Autodesk Inventor part; units mm, degrees
ref_plane "to_a_XY" through (0, 9.6037, 0) normal (0, 1, 0) x (1, 0, 0)
ref_plane "to_a_YZ" through (0, 9.6037, 0) normal (1, 0, 0) x (0, 0, -1)
ref_plane "to_a_ZX" through (0, 9.6037, 0) normal (0, 0, -1) x (0, 1, 0)
sketch "Sketch_1" plane through (0, 0, 0) normal (0, 0, 1) x (1, 0, 0)
  line L0 (0, 0) -> (0, 20.574)
  line L1 (0, 20.574) -> (2.6561, 20.574)
  arc A0 (5.5506, 18.0111) -> (2.6561, 20.574) centre (0.9891, 15.7753) ccw
  line L2 (5.5506, 18.0111) -> (5.5506, 17.2237)
  line L3 (5.5506, 17.2237) -> (2.3752, 17.2237)
  line L4 (2.3752, 17.2237) -> (2.3752, 10.414)
  line L5 (2.3752, 10.414) -> (3.175, 10.414)
  line L6 (3.175, 10.414) -> (3.175, 0.7557)
  line L7 (3.175, 0.7557) -> (2.4194, 0)
  line L8 (2.4194, 0) -> (0, 0)
  line L9 (0, 0) -> (0, 20.574)
revolve "Revolution1" add sketch "Sketch_1" angle 360 about axis through (0, 0, 0) along (0, -1, 0)
thread "Thread1"
sketch "Sketch_2" plane through (0, 20.574, 0) normal (0, 1, 0) x (1, 0, 0)
  line L0 (-7.62, 7.62) -> (-7.62, -7.62)
  line L1 (-7.62, -7.62) -> (7.62, -7.62)
  line L2 (7.62, -7.62) -> (7.62, 7.62)
  line L3 (7.62, 7.62) -> (-7.62, 7.62)
  line L4 (-2.3752, 6.35) -> (-2.3752, -6.35)
  line L5 (-2.3752, -6.35) -> (2.3752, -6.35)
  line L6 (2.3752, -6.35) -> (2.3752, 6.35)
  line L7 (2.3752, 6.35) -> (-2.3752, 6.35)
extrude "Extrusion1" cut sketch "Sketch_2" along normal mid plane 10.16
sketch "Sketch_3" plane through (0, 20.574, 0) normal (0, 1, 0) x (1, 0, 0)
  line L0 (-1.9814, -1.144) -> (0, -2.288)
  line L1 (0, -2.288) -> (1.9814, -1.144)
  line L2 (1.9814, -1.144) -> (1.9814, 1.144)
  line L3 (1.9814, 1.144) -> (0, 2.288)
  line L4 (0, 2.288) -> (-1.9814, 1.144)
  line L5 (-1.9814, 1.144) -> (-1.9814, -1.144)
extrude "Extrusion2" cut sketch "Sketch_3" against normal blind 2.2098
ref_plane "to_a_XY" through (0, 9.6037, 0) normal (0, 1, 0) x (1, 0, 0)
ref_plane "to_a_YZ" through (0, 9.6037, 0) normal (1, 0, 0) x (0, 0, -1)
ref_plane "to_a_ZX" through (0, 9.6037, 0) normal (0, 0, -1) x (0, 1, 0)
properties part number "2059_screw"
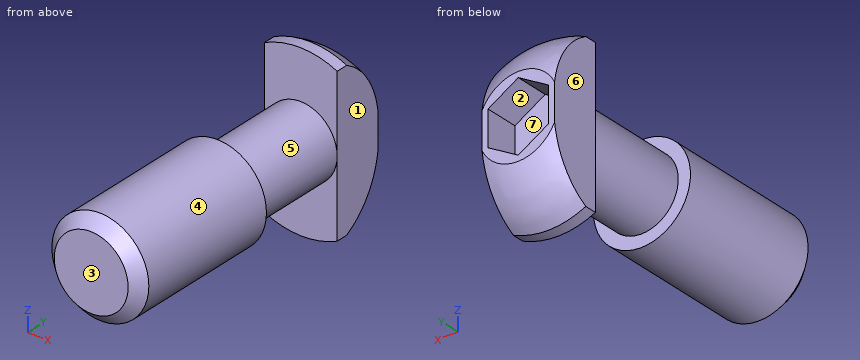
The listing builds one solid part. Answer for the finished solid, in the listing's coordinates (mm). Face numbers are marked on the shaded views. A direction names the side the tool comes from. Give positions to 0.01 mm unless a question says otherwise; leave off trailing zeros. Order: outer loops, then holes, each group sorted by start corner. A loop starts at its lowest first (then second) coordinate and runs counter-clockwise, first axis right, second up. Notation, with made-up numbers: (73.5, 74.5) - (88.5, 74.5) arc R19 cw to (88.5, 82.5) - close; hole circle Ø4 at (84.5, -9.75). An arc over 180 degrees is marked (long way). One line per item, written item: value. Start each with the question number.
1) A tool of negligible diameter and unlimited length cuts with its end or side. For the marked faces 1, 2, 3 and 4, from which of +Z, -Z, +X, -X, +Y, -Y can it reach the whole face along a straight path? Write none if from no direction.
2) Find the intervals of material crossed by L1, parallel to Y at x = 1.25, z = -1; L2, parallel to X at y = 17.5, z = -3.25; L3, parallel to Z at x = -1.5, y = 9.5, in increasing order.
3) Given pin 1 Ø1 at (x, y) = (2, 7.5) entering from +Z; pin 2 Ø1 at (x, z) = (0.5, 3) entering from -Y; pin 3 Ø1.8 at (y, z) = (19, -0.5) entering from +X, each flat-ended and moving along its own axis, determine where each tip first touches the part or whether it passes through.
4) The mould has two halves that part along Z. Classify the marked faces 5, 6 and 7: released by +Z, released by -Z, zero draft, split by the parting line, or undercut.
5) A cutting plane is placed at C-C on y = 3.5. Give the vertices of the cut face in (x, z) (3 decimals).
6) A cutting plane is placed at A-A on y = 17.5. Give the vertices of the cut face in (x, z), then the cut area to 3 significant figures.
7) A cutting plane is placed at B-B on y = 11. Give the vertices of the cut face in (x, z).
Answer sheet:
1. face 1: +Z, -Z, +X, +Y
1. face 2: +Y
1. face 3: +Z, -Z, +X, -X, -Y
1. face 4: -Y
2. L1: y = 0 to 18.36
2. L2: x = -2.38 to 2.38
2. L3: z = -2.8 to 2.8
3. pin 1: stops at z = 2.8
3. pin 2: stops at y = 0.12
3. pin 3: stops at x = 2.38
4. face 5: split by the parting line
4. face 6: zero draft
4. face 7: undercut
5. outline: circle Ø6.35 at (0, 0)
6. outline: (-2.38, -5.02) arc R5.55 ccw to (2.38, -5.02) - (2.38, 5.02) arc R5.55 ccw to (-2.38, 5.02) - close
6. area: 51.1 mm2
7. outline: circle Ø4.75 at (0, 0)
